Input: part model. Units: mm. Frame: model coordinates. Face numbers are marked on the shaded views. Give positions to 0.01 mm unless a question says otherwise; leave off trailing zeros. Loops run counter-clockwise (first coordinate to the right, second up) from the corner with the lowest first, then second, coordinate; pieces in that order, holes last. Notation, with made-up numbers: (60.25, -11) -> (83.25, -11) arc R23 cw to (83.25, 7) -> close; hole circle Ø4 at (11, 77.5). An arc over 180 degrees is marked (long way). Use CSV: the item, a comma, the result in double quotes.
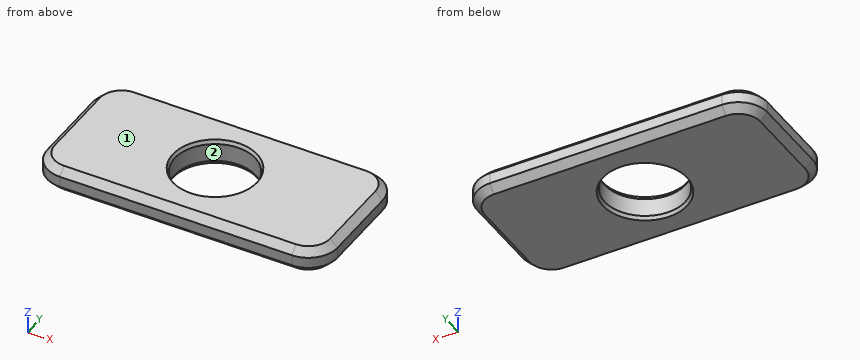
```python
from build123d import *

# Parameters (mm, degrees)
F0_R     = 11.1
F1_DEPTH = 7
F2_SIZE  = 2
F3_SIZE2 = 0.5
F3_SIZE  = 1


with BuildPart() as f1:
    # F0 (on Top) → F1 (new body)
    with BuildSketch(Plane.XY):
        with BuildLine():
            Line((-32, -19), (32, -19))
            ThreePointArc((32, -19), (37.6568542495, -16.6568542495), (40, -11))
            Line((40, -11), (40, 11))
            ThreePointArc((40, 11), (37.6568542495, 16.6568542495), (32, 19))
            Line((32, 19), (-32, 19))
            ThreePointArc((-32, 19), (-37.6568542495, 16.6568542495), (-40, 11))
            Line((-40, 11), (-40, -11))
            ThreePointArc((-40, -11), (-37.6568542495, -16.6568542495), (-32, -19))
        make_face()
        Circle(F0_R, mode=Mode.SUBTRACT)
    extrude(amount=F1_DEPTH)

    # F2
    f2_edges = [f1.edges().sort_by_distance(p)[0] for p in [
        (0, -19, 7),
        (0, -19, 0),
    ]]
    chamfer(f2_edges, length=F2_SIZE)

    # F3
    f3_edges = [f1.edges().sort_by_distance(p)[0] for p in [
        (-11.1, 0, 7),
        (-11.1, 0, 0),
    ]]
    f3_side = f1.faces().sort_by_distance((-11.1, 0, 3.5))[0]
    chamfer(f3_edges, length=F3_SIZE, length2=F3_SIZE2, reference=f3_side)


solid = f1.part
```
1) Ray query, line 1 (Y direction, x = 0, z = 2.05); line 2 (X direction, y = -6, z = 2.75); line 3 (X direction, y = -6.5, z = 0.75). Return the intervals inside material, ascending.
From the geometry:
line 1,"y = -19 to -11.1, 11.1 to 19"
line 2,"x = -40 to -9.34, 9.34 to 40"
line 3,"x = -38.75 to -9.15, 9.15 to 38.75"
2) Section query B-B (x = 0). Return loops of the section in (y, z).
From the geometry:
outline,"(-19, 2) -> (-17, 0) -> (-11.6, 0) -> (-11.1, 1) -> (-11.1, 6) -> (-11.6, 7) -> (-17, 7) -> (-19, 5) -> close; (11.1, 1) -> (11.6, 0) -> (17, 0) -> (19, 2) -> (19, 5) -> (17, 7) -> (11.6, 7) -> (11.1, 6) -> close"
3) Section query A-A (y = 0). Return loops of the section in (x, z), then the cut area to 3 significant figures.
From the geometry:
outline,"(-40, 2) -> (-38, 0) -> (-11.6, 0) -> (-11.1, 1) -> (-11.1, 6) -> (-11.6, 7) -> (-38, 7) -> (-40, 5) -> close; (11.1, 1) -> (11.6, 0) -> (38, 0) -> (40, 2) -> (40, 5) -> (38, 7) -> (11.6, 7) -> (11.1, 6) -> close"
area,"396 mm^2"
4) Mould query, pull axis Y, two halves, no side actions, for the marked faces 1 and 2. Classes: pulls with the +Y half, pulls with the -Y half, needs draft (parallel to the pull), parting line crosses it, or undercut.
From the geometry:
face 1,"needs draft"
face 2,"undercut"
5) Section query C-C (x = 16.5). Return loops of the section in (y, z), then the cut area to 3 significant figures.
From the geometry:
outline,"(-19, 2) -> (-17, 0) -> (17, 0) -> (19, 2) -> (19, 5) -> (17, 7) -> (-17, 7) -> (-19, 5) -> close"
area,"258 mm^2"
